Answer from the drawing. Dimensions are ordinates in mm from the lowest x, y and z of the part. Give positions to 0.01 mm unless a question says otherwise; leave off trailing zeros. Order: outer loops, then holes, each group sorted by start corner. A loop starts at its lowest first (then second) coordinate and runs counter-clockwise, first axis right, second up. Notation, with made-up numbers: (-21, 74) -> (-7, 74) arc R16 ccw to (-7, 91) -> close; hole circle Ø1 at (47.25, 52). An arc over 180 degrees is marked (long way). Answer as a JSON object with one key per item and string values. Group by question number.
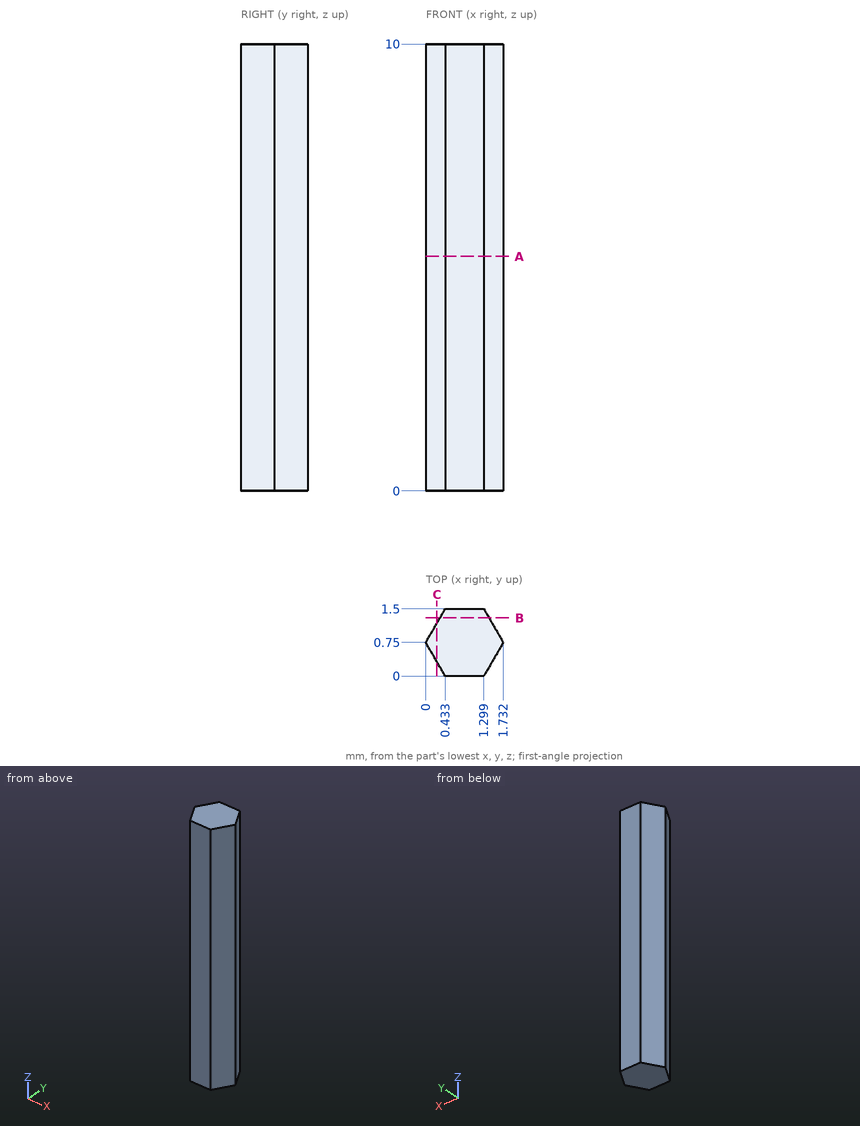
(1) Find the intervals of material crossed by line 1 along X through (y, z) = (0.8, 7.25); line 2 along Y through (x, z) = (1.6, 4.25); line 3 along X through (y, z) = (1.45, 1), in increasing order. Write a range as [from, to].
(2) A cutting plane is placed at A-A (z = 5.25). Determine the outline of the cut face in (x, y), and give its area (3 significant figures).
(3) A cutting plane is placed at B-B (y = 1.3). Determine the outline of the cut face in (x, z), and give its area (3 significant figures).
(4) A cutting plane is placed at C-C (x = 0.25). Determine the outline of the cut face in (y, z).
Check sheet entries:
{
 "1": {"line 1": "x = [0.03, 1.7]", "line 2": "y = [0.52, 0.98]", "line 3": "x = [0.4, 1.33]"},
 "2": {"outline": "(0, 0.75) -> (0.43, 0) -> (1.3, 0) -> (1.73, 0.75) -> (1.3, 1.5) -> (0.43, 1.5) -> close", "area": "1.95 mm2"},
 "3": {"outline": "(0.32, 0) -> (1.41, 0) -> (1.41, 10) -> (0.32, 10) -> close", "area": "11.0 mm2"},
 "4": {"outline": "(0.32, 0) -> (1.18, 0) -> (1.18, 10) -> (0.32, 10) -> close"}
}
